The model under review builds one solid part; all positions refer to its coordinate system, in mm. A direction names the side the tool comes from. Round coordinates to 2 decimals unless told otherwise and drop trailing zeros. Write each loop counter-clockwise with the first axis right and the second up, starting at its lowest first coordinate (ties: lowest second). Pieces come first, ordered by that corner, then holes. Notation, with made-up numbers: M -10.75,-18 L 44.25,-18 A38 ccw 44.25,20 Z; hole C -35,89.5 d11. An arc over 180 degrees is marked long. One line per item, written item: value. Start each with the question number.
1) Tool access review of faces 1 (the face through (294, 96, 2)), 2 (the face through (210, 96, 0)), 3 (the face through (127, 96, 2)): name each direction out of +Z, -Z, +X, -X, +Y, -Y from which nothing blocks a thin tool from reaching the whole face with its end or side.
2) Wall thickness on probe 1 along X at (y, z) = (75, 2.7); probe 2 along Z at (x, y) = (136, 125); probe 3 along X at (y, z) = (37.5, 1.4): over which ranges is each line inside the solid? List them lowest first.
3) Take a section at A-A, the plane z = 0.9. Write out the cut boundary in (x, y), and give its area (3 significant figures).
4) For P1, Ø1.6, axis at y = 20, z = 1.5, coming from the -X side; P2, Ø7, axis at x = 296.5, y = 58.5, coming from the +Z side; P3, Ø1, axis at x = 125, z = 1, coming from the +Y side, all flat-tipped, find the tip position at first contact; note any pin that passes through.
5) Take a section at C-C, the plane x = 290. Write out the cut boundary in (y, z).
6) Take a section at B-B, the plane y = 160. Write out the cut boundary in (x, z).
7) Take a section at D-D, the plane y = 44. Write out the cut boundary in (x, z), and give its area (3 significant figures).
from build123d import *

# Parameters (mm, degrees)
PAD_DEPTH    = 2
SKETCH004_W  = 144
SKETCH004_H  = 190
PAD001_DEPTH = 6


with BuildPart() as part:
    # Sketch001 → Pad (new body)
    with BuildSketch(Plane.XY):
        Polygon((136, 0), (286, 0), (286, 41), (306, 41), (306, 149), (286, 149), (286, 190), (136, 190), (136, 149), (116, 149), (116, 41), (136, 41), align=None)
    extrude(amount=PAD_DEPTH)

    # Sketch004 → Pad001 (join)
    with BuildSketch(Plane.XY):
        with Locations((211, 95)):
            Rectangle(SKETCH004_W, SKETCH004_H)
    extrude(amount=PAD001_DEPTH)


solid = part.part
Checked values:
1. face 1: +Z, +X, +Y, -Y
1. face 2: -Z, +X, -X, +Y, -Y
1. face 3: +Z, -X, +Y, -Y
2. probe 1: x = 139 to 283
2. probe 2: z = 0 to 2
2. probe 3: x = 136 to 286
3. outline: M 116,41 L 136,41 L 136,0 L 286,0 L 286,41 L 306,41 L 306,149 L 286,149 L 286,190 L 136,190 L 136,149 L 116,149 Z
3. area: 32,800 mm2
4. P1: stops at x = 136
4. P2: stops at z = 2
4. P3: stops at y = 149
5. outline: M 41,0 L 149,0 L 149,2 L 41,2 Z
6. outline: M 136,0 L 286,0 L 286,2 L 283,2 L 283,6 L 139,6 L 139,2 L 136,2 Z
7. outline: M 116,0 L 306,0 L 306,2 L 283,2 L 283,6 L 139,6 L 139,2 L 116,2 Z
7. area: 956 mm2
